```python
from build123d import *

# Parameters (mm, degrees)
SKETCH1_W           = 8
SKETCH1_H           = 5
BOSS_EXTRUDE1_DEPTH = 3
SKETCH2_W           = 3
SKETCH2_H           = 5
BOSS_EXTRUDE2_DEPTH = 5
SKETCH3_R           = 1.5
CUT_EXTRUDE1_DEPTH  = 5
SKETCH4_R           = 1.5
CUT_EXTRUDE2_DEPTH  = 5


with BuildPart() as part:
    # Sketch1 → Boss-Extrude1 (new body)
    with BuildSketch(Plane(origin=(0, 0, 0), x_dir=(1, 0, 0), z_dir=(0, 1, 0))):
        Rectangle(SKETCH1_W, SKETCH1_H)
    extrude(amount=BOSS_EXTRUDE1_DEPTH)

    # Sketch2 → Boss-Extrude2 (add)
    with BuildSketch(Plane(origin=(0, 3, 0), x_dir=(1, 0, 0), z_dir=(0, 1, 0))):
        with Locations((2.5, 0)):
            Rectangle(SKETCH2_W, SKETCH2_H)
    extrude(amount=BOSS_EXTRUDE2_DEPTH)

    # Sketch3 → Cut-Extrude1 (cut)
    with BuildSketch(Plane(origin=(0, 3, 0), x_dir=(1, 0, 0), z_dir=(0, 1, 0))):
        with Locations(Location((-1.5, 0, 0), (0, 0, 270))):
            Circle(SKETCH3_R)
    extrude(amount=-CUT_EXTRUDE1_DEPTH, mode=Mode.SUBTRACT)

    # Sketch4 → Cut-Extrude2 (cut)
    with BuildSketch(Plane.ZY.offset(-1)):
        with Locations((0, 5.5)):
            Circle(SKETCH4_R)
    extrude(amount=-CUT_EXTRUDE2_DEPTH, mode=Mode.SUBTRACT)


solid = part.part
```
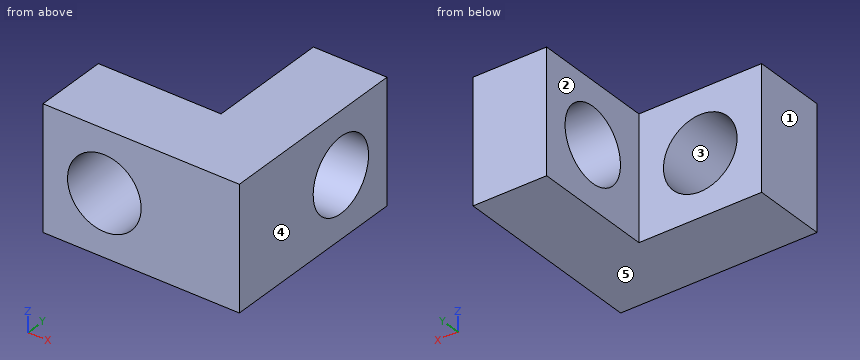
Part model, mm, in its own coordinate system. Face numbers are marked on the shaded views. A direction names the side the tool comes from. Coordinates: 2 decimals unless noted, no trailing zeros. Order: outer loops, then holes, each group sorted by start corner. A loop starts at its lowest first (then second) coordinate and runs counter-clockwise, first axis right, second up. Notation, with made-up numbers: (63, 4) - (94, 4) arc R27 ccw to (94, 27) - close; hole circle Ø6 at (-22.5, 68). An arc over 180 degrees is marked (long way). Return JSON: item names as keys, results as strings. Group by question number.
Item 1: Cut at A-A (x = -1.5). List the corners of the cut face in (y, z).
Item 2: Drill centre lines: probe 1 along X at (y, z) = (1.25, -0.1); probe 2 along X at (y, z) = (7, 0.9); probe 3 along Y at (x, z) = (2.75, -0.3). Where is each one in solid material? Low to high. Write a range as from..to.
Item 3: Pull direction Z, two halves, no side cores. Call the marked faces 3, 4 and 5: pulls with the +Z half, pulls with the -Z half, needs draft (parallel to the pull), parting line crosses it, or undercut.
Item 4: Which spindle directions (+Z, -Z, +X, -X, +Y, -Y) get a long thin tool onto all of the face, cutting with end or side? Do the marked faces 1 and 2. Say none if no direction does.
Item 5: Cut at D-D (x = 3.25). List the corners of the cut face in (y, z).
Item 6: Cut at C-C (z = 0.9). List the corners of the cut face in (x, y), plus the area to 3 significant figures.
Item 7: Cut at B-B (y = 5.5). List the corners of the cut face in (x, z), plus the area to 3 significant figures.
Item 8: Pin check, flat tips, straight feed: pin 1 (1.8 mm diameter, centred on x = -1.5, z = 0, fed in from -Y); pin 2 (2 mm diameter, centred on y = 5.5, z = 1.5, fed in from -X); pin 3 (2.5 mm diameter, centred on x = -2.5, z = -0.5, fed in from +Y). Stop position of each tip, or through.
Check values:
{
 "1": {"outline": "(0, -2.5) - (3, -2.5) - (3, -1.5) - (0, -1.5) - close; (0, 1.5) - (3, 1.5) - (3, 2.5) - (0, 2.5) - close"},
 "2": {"probe 1": "x = -4..-3, 0..4", "probe 2": "x = 1..4", "probe 3": "y = 0..4.03, 6.97..8"},
 "3": {"face 3": "undercut", "face 4": "needs draft", "face 5": "pulls with the -Z half"},
 "4": {"face 1": "+Z, -Z, -X, +Y, -Y", "face 2": "+Z, -Z, -X, +Y"},
 "5": {"outline": "(0, -2.5) - (8, -2.5) - (8, 2.5) - (0, 2.5) - close; hole circle Ø3 at (5.5, 0)"},
 "6": {"outline": "(-4, 0) - (-2.7, 0) - (-2.7, 3) - (-4, 3) - close; (-0.3, 0) - (4, 0) - (4, 4.3) - (1, 4.3) - (1, 3) - (-0.3, 3) - close; (1, 6.7) - (4, 6.7) - (4, 8) - (1, 8) - close", "area": "24.6 mm2"},
 "7": {"outline": "(1, -2.5) - (4, -2.5) - (4, -1.5) - (1, -1.5) - close; (1, 1.5) - (4, 1.5) - (4, 2.5) - (1, 2.5) - close", "area": "6.00 mm2"},
 "8": {"pin 1": "passes through", "pin 2": "stops at x = 1", "pin 3": "stops at y = 3"}
}
